```python
from build123d import *
from build123d.topology import SkipClean

# Parameters (mm, degrees)
SKETCH_1_R          = 10
EXTRUDE_1_DEPTH     = 2
EXTRUDE_2_DEPTH     = 3
SKETCH_3_R          = 3.2
CUT_EXTRUDE_1_DEPTH = 3
EXTRUDE_3_DEPTH     = 1
SKETCH_6_R          = 7
SKETCH_6_R_2        = 3.2
EXTRUDE_4_DEPTH     = 5
SKETCH_7_W          = 8.062767077
SKETCH_7_H          = 6
EXTRUDE_5_DEPTH     = 5
SKETCH_8_R          = 1.5
CUT_EXTRUDE_3_DEPTH = 20.006577809
CUT_EXTRUDE_4_DEPTH = 5
FILLET_7_R          = 1.5
EXTRUDE_6_DEPTH     = 3
EXTRUDE_START       = -2
SKETCH_12_R         = 3.2
EXTRUDE_7_DEPTH     = 2
FILLET_8_R          = 3
EXTRUDE_8_DEPTH     = 3.5
SKETCH_14_R         = 1.6
CUT_EXTRUDE_5_DEPTH = 22.640009284


with BuildPart() as part:
    # 草图1 → 凸台-拉伸1 (new body)
    with BuildSketch(Plane.XY):
        Circle(SKETCH_1_R)
    extrude(amount=EXTRUDE_1_DEPTH)

    # 草图2 → 凸台-拉伸2 (add)
    with SkipClean():  # the faces are left unmerged after this step: merging them gives an invalid solid
        with BuildSketch(Plane.XY.offset(2)):
            with BuildLine():
                Line((3.376388603, -5.2), (8.541662602, -5.2))
                ThreePointArc((8.541662602, -5.2), (6.403471398, -7.680856336), (3.578411207, -9.337824866))
                ThreePointArc((3.578411207, -9.337824866), (-0.425231333, -9.990954825), (-4.358898944, -9))
                ThreePointArc((-4.358898944, -9), (-6.724293423, -7.401613199), (-8.541662602, -5.2))
                Line((-8.541662602, -5.2), (-3.376388603, -5.2))
                ThreePointArc((-3.376388603, -5.2), (0, -6.2), (3.376388603, -5.2))
            make_face()
            with BuildLine():
                Line((-4.2, 5.2), (-8.541662602, 5.2))
                ThreePointArc((-8.541662602, 5.2), (-6.658968745, 7.460438007), (-4.2, 9.075241044))
                Line((-4.2, 9.075241044), (-4.2, 5.2))
            make_face()
            with BuildLine():
                Line((5.7, 5.2), (8.541662602, 5.2))
                ThreePointArc((8.541662602, 5.2), (7.278803227, 6.857041897), (5.7, 8.216446921))
                Line((5.7, 8.216446921), (5.7, 5.2))
            make_face()
        extrude(amount=EXTRUDE_2_DEPTH)

    # 草图3 → 切除-拉伸1 (cut)
    with SkipClean():  # the faces are left unmerged after this step: merging them gives an invalid solid
        with BuildSketch(Plane.XY.offset(2)):
            Circle(SKETCH_3_R)
        extrude(amount=-CUT_EXTRUDE_1_DEPTH, mode=Mode.SUBTRACT)

    # 草图5 → 凸台-拉伸3 (add)
    with SkipClean():  # the faces are left unmerged after this step: merging them gives an invalid solid
        with BuildSketch(Plane(origin=(0, 0, 0), x_dir=(-1, 0, 0), z_dir=(0, 0, -1))):
            with BuildLine():
                Line((-3.5, 6.062177826), (-3.5, 3.2))
                Line((-3.5, 3.2), (3.5, 3.2))
                Line((3.5, 3.2), (3.5, 6.062177826))
                ThreePointArc((3.5, 6.062177826), (0, 7), (-3.5, 6.062177826))
            make_face()
        extrude(amount=EXTRUDE_3_DEPTH)

    # 草图6 → 凸台-拉伸4 (add)
    with SkipClean():  # the faces are left unmerged after this step: merging them gives an invalid solid
        with BuildSketch(Plane(origin=(0, 0, -1), x_dir=(-1, 0, 0), z_dir=(0, 0, -1))):
            with Locations(Location((0, 0, 0), (0, 0, 120))):
                Circle(SKETCH_6_R)
            with Locations(Location((0, 0, 0), (0, 0, 180))):
                Circle(SKETCH_6_R_2, mode=Mode.SUBTRACT)
        extrude(amount=EXTRUDE_4_DEPTH)

    # 草图7 → 凸台-拉伸5 (add)
    with SkipClean():  # the faces are left unmerged after this step: merging them gives an invalid solid
        with BuildSketch(Plane(origin=(0, 0, -6), x_dir=(-1, 0, 0), z_dir=(0, 0, -1))):
            with Locations((8.468616461, 0)):
                Rectangle(SKETCH_7_W, SKETCH_7_H)
        extrude(amount=-EXTRUDE_5_DEPTH)

    # 草图8 → 切除-拉伸3 (cut, through all)
    with SkipClean():  # the faces are left unmerged after this step: merging them gives an invalid solid
        with BuildSketch(Plane(origin=(0, 3, 0), x_dir=(1, 0, 0), z_dir=(0, 1, 0))):
            with Locations(Location((-9.5, 3.5, 0), (0, 0, 270))):
                Circle(SKETCH_8_R)
        extrude(amount=-CUT_EXTRUDE_3_DEPTH, mode=Mode.SUBTRACT)

    # 草图9 → 切除-拉伸4 (cut)
    with SkipClean():  # the faces are left unmerged after this step: merging them gives an invalid solid
        with BuildSketch(Plane(origin=(0, 0, -6), x_dir=(-1, 0, 0), z_dir=(0, 0, -1))):
            Polygon((0, 0), (0, 1), (12.5, 1), (12.5, -1), (0, -1), align=None)
        extrude(amount=-CUT_EXTRUDE_4_DEPTH, mode=Mode.SUBTRACT)

    # 圆角7
    fillet_7_edges = [part.edges().sort_by_distance(p)[0] for p in [
        (-12.5, 2, -1),
        (-12.5, -2, -1),
        (-12.5, -2, -6),
        (-12.5, 2, -6),
    ]]
    fillet(fillet_7_edges, radius=FILLET_7_R)

    # 草图10 → 凸台-拉伸6 (add)
    with BuildSketch(Plane(origin=(0, 0, -6), x_dir=(-1, 0, 0), z_dir=(0, 0, -1))):
        with BuildLine():
            Line((2, 6.708203932), (2, 2.497999199))
            ThreePointArc((2, 2.497999199), (0, 3.2), (-2, 2.497999199))
            Line((-2, 2.497999199), (-2, 6.708203932))
            ThreePointArc((-2, 6.708203932), (0, 7), (2, 6.708203932))
        make_face()
    extrude(amount=EXTRUDE_6_DEPTH)

    # 草图12 → 凸台-拉伸7 (add)
    with BuildSketch(Plane(origin=(0, 0, -9), x_dir=(-1, 0, 0), z_dir=(0, 0, -1)).offset(EXTRUDE_START)):
        with Locations(Location((0, 0, 0), (0, 0, 180))):
            Circle(SKETCH_12_R)
    extrude(amount=EXTRUDE_7_DEPTH)

    # 圆角8
    fillet_8_edges = [part.edges().sort_by_distance(p)[0] for p in [
        (0, 7, -9),
    ]]
    fillet(fillet_8_edges, radius=FILLET_8_R - 0.0001)  # a hair under: the kernel refuses the full size

    # 草图13 → 凸台-拉伸8 (add)
    with BuildSketch(Plane.XY.offset(5)):
        with BuildLine():
            Line((3.376388603, -5.2), (8.541662602, -5.2))
            ThreePointArc((8.541662602, -5.2), (0, -10), (-8.541662602, -5.2))
            Line((-8.541662602, -5.2), (-3.376388603, -5.2))
            ThreePointArc((-3.376388603, -5.2), (0, -6.2), (3.376388603, -5.2))
        make_face()
    extrude(amount=EXTRUDE_8_DEPTH)

    # 草图14 → 切除-拉伸5 (cut, through all)
    with BuildSketch(Plane(origin=(0, -5.2, 0), x_dir=(1, 0, 0), z_dir=(0, 1, 0))):
        with Locations(Location((4.5, -6, 0), (0, 0, 270))):
            Circle(SKETCH_14_R)
        with Locations(Location((-4.5, -6, 0), (0, 0, 270))):
            Circle(SKETCH_14_R)
    extrude(amount=-CUT_EXTRUDE_5_DEPTH, mode=Mode.SUBTRACT)


solid = part.part
```
Work out the finished part from the listing and answer in its coordinate system (mm). A direction names the side the tool comes from. Give positions to 0.01 mm unless a question says otherwise; leave off trailing zeros. Loops run counter-clockwise (first coordinate to the right, second up) from the corner with the lowest first, then second, coordinate; pieces in that order, holes last. Notation, with made-up numbers: (3, -15.75) -> (11, -15.75) arc R24 cw to (11, 20.25) -> close; hole circle Ø5 at (-8, -10.5). An arc over 180 degrees is marked (long way). Write item = value, one per line. Start each with the question number.
(1) Find section D-D on y = -4.5. Give the vertices of the cut face in (x, z), and give its area (3 significant figures).
(2) Find the intervals of material crossed by probe 1 along Y at (x, z) = (-6.5, -2); probe 2 along Y at (x, z) = (0, 1.6); probe 3 along Z at (x, y) = (4.5, -6.3), in increasing order. Write a range as from..to.
(3) The mould has two halves that part along Y. Classify faces 1 (the flat face through (5.7, 7, 3)), 2 (the flat face through (0, 3.2, -0.5)), 3 (the flat face through (-7, -5.2, 5)): +Y half, -Y half, draft (parallel to the pull), parting line (faces both ways), or undercut.
(4) Which of the six approach directions +Z, -Z, +X, -X, +Y, -Y give full straight-line access (tool end or side, diameter ignored) to faces 4 (the flat face through (-2, 4, -7)), 5 (the flat face through (7, 6, 5)), 6 (the flat face through (2, 5, -7)), 7 (the flat face through (2, -3, -6))?
(5) Find section B-B on y = 0. Give the vertices of the cut face in (x, z).
(6) Find section A-A on z = -3.5. Give the vertices of the cut face in (x, y), and give its area (3 significant figures).
(7) Given pin 1 Ø3.5 at (y, z) = (4.5, -7) entering from -X; pin 2 Ø2 at (y, z) = (7, 5.5) entering from +X; pin 3 Ø3 at (x, y) = (-6, 7.5) entering from +Z, each flat-ended and moving along its own axis, determine where each tip first touches the part or whether it passes through.
(8) Find section C-C on x = -9.5. Give the vertices of the cut face in (y, z), and give its area (3 significant figures).
From the geometry:
q1.outline = (-8.93, 0) -> (8.93, 0) -> (8.93, 2) -> (-8.93, 2) -> close; (-5.36, -6) -> (5.36, -6) -> (5.36, -1) -> (-5.36, -1) -> close
q1.area = 89.3 mm^2
q2.probe_1 = -3..-1, 1..3
q2.probe_2 = -10..-3.2, 3.2..10
q2.probe_3 = 0..4.4, 7.6..8.5
q3.face_1 = draft
q3.face_2 = -Y half
q3.face_3 = undercut
q4.face_4 = -Z, -X, +Y
q4.face_5 = +Z, +X, -X, +Y
q4.face_6 = -Z, +X, +Y
q4.face_7 = -Z, +X, -Y
q5.outline = (-10, 0) -> (-3.2, 0) -> (-3.2, 2) -> (-10, 2) -> close; (-3.2, -9) -> (3.2, -9) -> (3.2, -7) -> (-3.2, -7) -> close; (3.2, -6) -> (7, -6) -> (7, -1) -> (3.2, -1) -> close; (3.2, 0) -> (10, 0) -> (10, 2) -> (3.2, 2) -> close
q6.outline = (-12.5, -3) -> (-11, -3) -> (-11, -1) -> (-12.5, -1) -> close; (-12.5, 1) -> (-11, 1) -> (-11, 3) -> (-12.5, 3) -> close; (-8, -3) -> (-6.32, -3) arc R7 ccw (long way) to (-6.32, 3) -> (-8, 3) -> (-8, 1) -> (-3.04, 1) arc R3.2 cw (long way) to (-3.04, -1) -> (-8, -1) -> close
q6.area = 125 mm^2
q7.pin_1 = -6.29
q7.pin_2 = 7.9
q7.pin_3 = 5
q8.outline = (-3.12, 0) -> (3.12, 0) -> (3.12, 2) -> (-3.12, 2) -> close; (-3, -6) -> (-1, -6) -> (-1, -5) -> (-3, -5) -> close; (-3, -2) -> (-1, -2) -> (-1, -1) -> (-3, -1) -> close; (1, -6) -> (3, -6) -> (3, -5) -> (1, -5) -> close; (1, -2) -> (3, -2) -> (3, -1) -> (1, -1) -> close
q8.area = 20.5 mm^2
